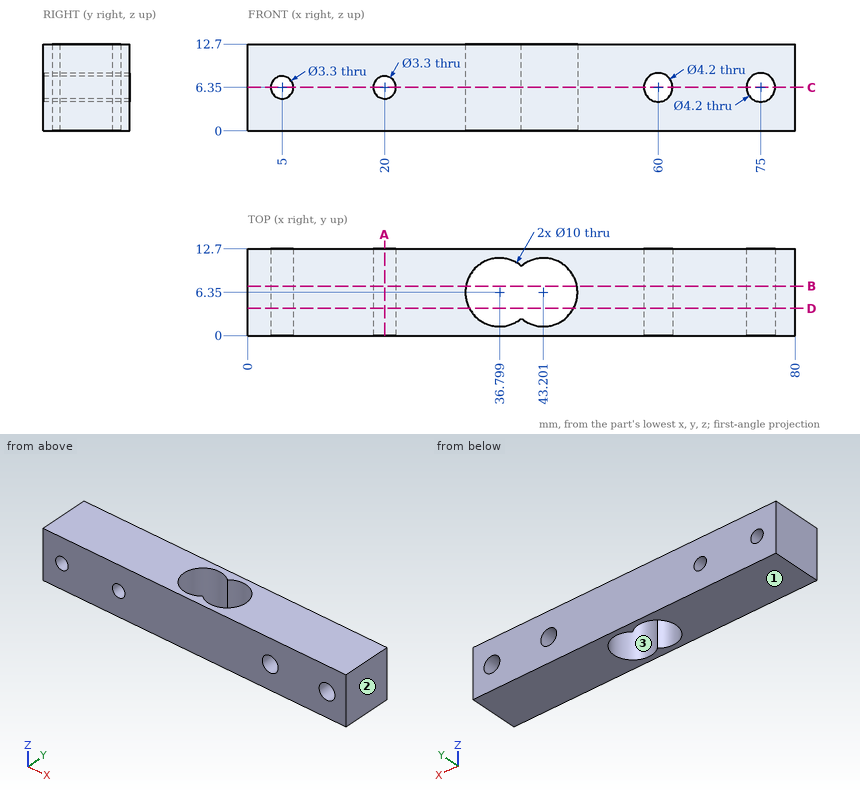
Design review of the part shown in the three views and the two pictorial views. Dimensions are in mm from the part's minimum x, y and z. Round coordinates to 2 decimals unless told otherwise and drop trailing zeros. Loops run counter-clockwise (first coordinate to the right, second up) from the corner with the lowest first, then second, coordinate; pieces in that order, holes last.
1) Wall thickness on line 1 along Z through (x, y) = (60, 4.25); line 2 along X through (y, z) = (9.75, 6); line 3 along X through (y, z) = (6.75, 11.5) (1 decimal): over which ranges is each line inside the solid? List them lowest first.
Values follow:
line 1: z = 0 to 4.25, 8.45 to 12.7
line 2: x = 0 to 3.39, 6.61 to 18.39, 21.61 to 33.13, 46.87 to 57.93, 62.07 to 72.93, 77.07 to 80
line 3: x = 0 to 31.8, 48.2 to 80
2) Consider section C-C on z = 6.35. State the section outline as (x, y) points.
Values follow:
outline: (0, 0) - (3.35, 0) - (3.35, 12.7) - (0, 12.7) - close; (6.65, 0) - (18.35, 0) - (18.35, 12.7) - (6.65, 12.7) - close; (21.65, 0) - (57.9, 0) - (57.9, 12.7) - (21.65, 12.7) - close; (62.1, 0) - (72.9, 0) - (72.9, 12.7) - (62.1, 12.7) - close; (77.1, 0) - (80, 0) - (80, 12.7) - (77.1, 12.7) - close; hole (40, 2.51) arc R5 ccw (long way) to (40, 10.19) arc R5 ccw (long way) to start
3) The part is to be moulded in two halves that separate along X. For the marked faces 1, 2 and 3, say which applies: pulls with the +X half, pulls with the -X half, needs draft (parallel to the pull), parting line crosses it, or undercut.
Values follow:
face 1: needs draft
face 2: pulls with the +X half
face 3: undercut
4) Clearance check with flat-ended pins moving along their axes: P1, Ø3, axis at x = 20, z = 6.35, coming from the -Y side; P2, Ø5, axis at x = 60, z = 6.35, coming from the -Y side. State where each tip first meets the part, or that it passes through.
Values follow:
P1: passes through
P2: stops at y = 0
5) Consider section D-D on y = 4. State the section outline as (x, z) points.
Values follow:
outline: (0, 0) - (32.39, 0) - (32.39, 12.7) - (0, 12.7) - close; (47.61, 0) - (80, 0) - (80, 12.7) - (47.61, 12.7) - close; hole circle Ø3.3 at (5, 6.35); hole circle Ø3.3 at (20, 6.35); hole circle Ø4.2 at (60, 6.35); hole circle Ø4.2 at (75, 6.35)
6) Consider section B-B on y = 7.25. State the section outline as (x, z) points.
Values follow:
outline: (0, 0) - (31.88, 0) - (31.88, 12.7) - (0, 12.7) - close; (48.12, 0) - (80, 0) - (80, 12.7) - (48.12, 12.7) - close; hole circle Ø3.3 at (5, 6.35); hole circle Ø3.3 at (20, 6.35); hole circle Ø4.2 at (60, 6.35); hole circle Ø4.2 at (75, 6.35)
7) Consider section A-A on x = 20. State the section outline as (y, z) points, then the cut area to 3 significant figures.
Values follow:
outline: (0, 0) - (12.7, 0) - (12.7, 4.7) - (0, 4.7) - close; (0, 8) - (12.7, 8) - (12.7, 12.7) - (0, 12.7) - close
area: 119 mm2
